Can you work these out from the model? Positions are in its coordinate system, mm. Face numbers are marked on the shaded views. A direction names the side the tool comes from. Coordinates: 2 decimals unless noted, no trailing zeros. Order: outer loops, then holes, each group sorted by start corner. A loop starts at its lowest first (then second) coordinate and runs counter-clockwise, first axis right, second up. Notation, with made-up numbers: M 9.5,13 L 51.5,13 A4 cw 51.5,18 Z; hole C 29,9 d11. An arc over 180 degrees is marked long. Answer as CSV lines item,"result". Start each with the question number.
1. If we mould it in two halves opening along X, with no side actions, what happens to the marked faces 3, 4 and 5? For each: released by +X, released by -X, zero draft, split by the parting line, or undercut.
2. I need wall thicknesses on line 1 along Z through (x, y) = (15, 15.75); line 2 along X through (y, z) = (7.5, -2.5); line 3 along Y through (x, z) = (2, 0). Which ranges of each line are inside material? Lowest first, please. Write a range as from..to.
3. On a 3-axis mill with a long thin cutter (end or side, diameter ignored), from which of +Z, -Z, +X, -X, +Y, -Y can I reach the whole of each face in a straight line? I mean the marked faces 1 and 2. Say none if no direction works.
4. If we section it at B-B (z = 0): List the corners of the cut face in (x, y) for me, plus the area to 3 significant figures.
5. If we section it at A-A (y = 15.75): List the corners of the cut face in (x, z) for me, plus the area to 3 significant figures.
6. Will these pins go through, and if not, where does the flat tip stop? pin 1 (4.5 mm diameter, centred on x = 15, z = 12.5, fed in from +Y); pin 2 (8 mm diameter, centred on x = 16.5, y = 4.5, fed in from +Z); pin 3 (4 mm diameter, centred on x = -15, y = 17, fed in from +Z); pin 4 (6 mm diameter, centred on x = -13, y = 16.5, fed in from -Z).
7. If we section it at C-C (z = 12): List the corners of the cut face in (x, y) for me, plus the area to 3 significant figures.
8. If we section it at D-D (x = -15): List the corners of the cut face in (y, z) for me.
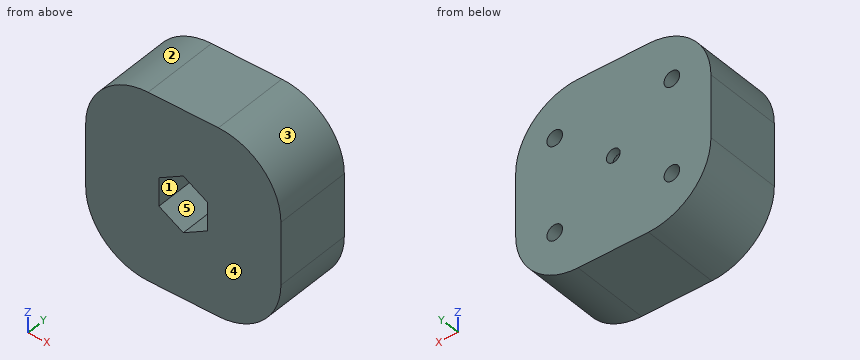
```python
from build123d import *

# Parameters (mm, degrees)
BOSS_EXTRUDE1_DEPTH = 18
SKETCH2_R           = 2
SKETCH2_R_2         = 1.75
BOSS_EXTRUDE3_DEPTH = 2
CUT_EXTRUDE1_START  = -10
SKETCH3_R           = 2
CUT_EXTRUDE1_DEPTH  = 10


with BuildPart() as part:
    # Sketch1 → Boss-Extrude1 (new body)
    with BuildSketch(Plane(origin=(0, 0, 0), x_dir=(1, 0, 0), z_dir=(0, 1, 0))):
        with BuildLine():
            Line((-9.000000373, 24.000000209), (9.000000373, 24.000000209))
            ThreePointArc((9.000000373, 24.000000209), (20.313708872, 19.313708708), (25.000000373, 8.000000209))
            Line((25.000000373, 8.000000209), (25.000000373, -8.000000209))
            ThreePointArc((25.000000373, -8.000000209), (20.313708872, -19.313708708), (9.000000373, -24.000000209))
            Line((9.000000373, -24.000000209), (-9.000000373, -24.000000209))
            ThreePointArc((-9.000000373, -24.000000209), (-20.313708872, -19.313708708), (-25.000000373, -8.000000209))
            Line((-25.000000373, -8.000000209), (-25.000000373, 8.000000209))
            ThreePointArc((-25.000000373, 8.000000209), (-20.313708872, 19.313708708), (-9.000000373, 24.000000209))
        make_face()
        Polygon((0, 7.216878365), (-6.25, 3.608439182), (-6.25, -3.608439182), (0, -7.216878365), (6.25, -3.608439182), (6.25, 3.608439182), align=None, mode=Mode.SUBTRACT)
    extrude(amount=BOSS_EXTRUDE1_DEPTH)

    # Sketch2 → Boss-Extrude3 (add)
    with BuildSketch(Plane(origin=(0, 18, 0), x_dir=(1, 0, 0), z_dir=(0, 1, 0))):
        with BuildLine():
            Line((-9.000000373, 24.000000209), (9.000000373, 24.000000209))
            ThreePointArc((9.000000373, 24.000000209), (20.313708872, 19.313708708), (25.000000373, 8.000000209))
            Line((25.000000373, 8.000000209), (25.000000373, -8.000000209))
            ThreePointArc((25.000000373, -8.000000209), (20.313708872, -19.313708708), (9.000000373, -24.000000209))
            Line((9.000000373, -24.000000209), (-9.000000373, -24.000000209))
            ThreePointArc((-9.000000373, -24.000000209), (-20.313708872, -19.313708708), (-25.000000373, -8.000000209))
            Line((-25.000000373, -8.000000209), (-25.000000373, 8.000000209))
            ThreePointArc((-25.000000373, 8.000000209), (-20.313708872, 19.313708708), (-9.000000373, 24.000000209))
        make_face()
        with Locations(Location((-14.999999943, 12.000001696, 0), (0, 0, 270))):
            Circle(SKETCH2_R, mode=Mode.SUBTRACT)
        with Locations(Location((14.999999943, 12.000001696, 0), (0, 0, 90))):
            Circle(SKETCH2_R, mode=Mode.SUBTRACT)
        with Locations(Location((14.999999943, -12.000001696, 0), (0, 0, 270))):
            Circle(SKETCH2_R, mode=Mode.SUBTRACT)
        with Locations(Location((-14.999999943, -12.000001696, 0), (0, 0, 90))):
            Circle(SKETCH2_R, mode=Mode.SUBTRACT)
        with Locations(Location((0, 0, 0), (0, 0, 270))):
            Circle(SKETCH2_R_2, mode=Mode.SUBTRACT)
    extrude(amount=BOSS_EXTRUDE3_DEPTH)

    # Sketch3 → Cut-Extrude1 (cut)
    with BuildSketch(Plane(origin=(0, 20, 0), x_dir=(1, 0, 0), z_dir=(0, 1, 0)).offset(CUT_EXTRUDE1_START)):
        with Locations(Location((-14.999999943, 12.000001696, 0), (0, 0, 270))):
            Circle(SKETCH3_R)
        with Locations(Location((14.999999943, 12.000001696, 0), (0, 0, 90))):
            Circle(SKETCH3_R)
        with Locations(Location((14.999999943, -12.000001696, 0), (0, 0, 270))):
            Circle(SKETCH3_R)
        with Locations(Location((-14.999999943, -12.000001696, 0), (0, 0, 90))):
            Circle(SKETCH3_R)
    extrude(amount=CUT_EXTRUDE1_DEPTH, mode=Mode.SUBTRACT)


solid = part.part
```
Solved:
1,face 3,"released by +X"
1,face 4,"zero draft"
1,face 5,"undercut"
2,line 1,"-22.83..-14, -10..10, 14..22.83"
2,line 2,"-25..-6.25, 6.25..25"
2,line 3,"18..20"
3,face 1,"-Y"
3,face 2,"+Z, -X, +Y, -Y"
4,outline,"M -25,0 L -6.25,0 L -6.25,18 L -1.75,18 L -1.75,20 L -25,20 Z; M 1.75,18 L 6.25,18 L 6.25,0 L 25,0 L 25,20 L 1.75,20 Z"
4,area,"768 mm²"
5,outline,"M -25,-8 A16 ccw -9,-24 L 9,-24 A16 ccw 25,-8 L 25,8 A16 ccw 9,24 L -9,24 A16 ccw -25,8 Z; hole C -15,-12 d4; hole C -15,12 d4; hole M -6.25,-3.61 L 0,-7.22 L 6.25,-3.61 L 6.25,3.61 L 0,7.22 L -6.25,3.61 Z; hole C 15,-12 d4; hole C 15,12 d4"
5,area,"1,990 mm²"
6,pin 1,"y = 20"
6,pin 2,"z = 23.61"
6,pin 3,"z = 23.49"
6,pin 4,"z = -23.97"
7,outline,"M -24.49,0 L 24.49,0 L 24.49,20 L 17,20 L 17,10 L 13,10 L 13,20 L -13,20 L -13,10 L -17,10 L -17,20 L -24.49,20 Z"
7,area,"900 mm²"
8,outline,"M 0,-22.83 L 20,-22.83 L 20,-14 L 10,-14 L 10,-10 L 20,-10 L 20,10 L 10,10 L 10,14 L 20,14 L 20,22.83 L 0,22.83 Z"
